Model file for the job. Use its own axes, mm. A direction names the side the tool comes from. Round coordinates to 2 decimals unless told otherwise and drop trailing zeros. Loops run counter-clockwise (first coordinate to the right, second up) from the corner with the lowest first, then second, coordinate; pieces in that order, holes last. Notation, with made-up numbers: (88, 9.5) - (143, 9.5) arc R10 cw to (143, 25.5) - close; hole circle Ø1 at (-25.5, 28.25). An arc over 180 degrees is marked (long way). Answer as a JSON object with one key per item and string values.
from build123d import *

# Parameters (mm, degrees)
F0_R     = 4.2591952999
F1_DEPTH = 2.286
F2_SIZE  = 1.016
F3_R     = 0.889
F4_SIZE  = 0.762
F5_SIZE  = 0.762


with BuildPart() as f1:
    # F0 (on Top) → F1 (new body)
    with BuildSketch(Plane.XY):
        Polygon((0, 14.6646975499), (-12.700000617, 21.9970463248), (-12.700000617, 7.3323487749), align=None)
        Polygon((12.700000617, 21.9970463248), (0, 14.6646975499), (12.700000617, 7.3323487749), align=None)
        Polygon((12.700000617, 7.3323487749), (0, 14.6646975499), (-12.700000617, 7.3323487749), (-12.700000617, -7.3323487749), (0, -14.6646975499), (12.700000617, -7.3323487749), align=None)
        Circle(F0_R, mode=Mode.SUBTRACT)
        Polygon((-12.700000617, -7.3323487749), (-12.700000617, 7.3323487749), (-25.400001234, 0), align=None)
        Polygon((-20.6551154208, 0), (-12.7952113226, 4.5379177469), (-12.7952113226, -4.5379177469), align=None, mode=Mode.SUBTRACT)
        Polygon((25.400001234, 0), (12.700000617, 7.3323487749), (12.700000617, -7.3323487749), align=None)
        Polygon((12.7952113226, -4.5379177469), (12.7952113226, 4.5379177469), (20.6551154208, 0), align=None, mode=Mode.SUBTRACT)
        Polygon((0, -14.6646975499), (-12.700000617, -7.3323487749), (-12.700000617, -21.9970463248), align=None)
        Polygon((12.700000617, -21.9970463248), (12.700000617, -7.3323487749), (0, -14.6646975499), align=None)
    extrude(amount=F1_DEPTH)

    # F2
    f2_edges = [f1.edges().sort_by_distance(p)[0] for p in [
        (-6.35, 18.330872, 2.286),
        (-12.700001, 14.664698, 2.286),
        (-19.050001, 3.666174, 2.286),
        (-19.050001, -3.666174, 2.286),
        (-12.700001, -14.664698, 2.286),
        (-6.35, -18.330872, 2.286),
        (6.35, -18.330872, 2.286),
        (12.700001, -14.664698, 2.286),
        (19.050001, -3.666174, 2.286),
        (19.050001, 3.666174, 2.286),
        (12.700001, 14.664698, 2.286),
        (6.35, 18.330872, 2.286),
    ]]
    chamfer(f2_edges, length=F2_SIZE)

    # F3
    f3_edges = [f1.edges().sort_by_distance(p)[0] for p in [
        (-4.259195, 0, 0),
        (-4.259195, 0, 2.286),
    ]]
    fillet(f3_edges, radius=F3_R)

    # F4
    f4_edges = [f1.edges().sort_by_distance(p)[0] for p in [
        (-6.35, -18.330872, 0),
        (6.35, -18.330872, 0),
        (12.700001, -14.664698, 0),
        (19.050001, -3.666174, 0),
        (19.050001, 3.666174, 0),
        (12.700001, 14.664698, 0),
        (6.35, 18.330872, 0),
        (-6.35, 18.330872, 0),
        (-12.700001, 14.664698, 0),
        (-19.050001, 3.666174, 0),
        (-19.050001, -3.666174, 0),
        (-12.700001, -14.664698, 0),
    ]]
    chamfer(f4_edges, length=F4_SIZE)

    # F5
    f5_edges = [f1.edges().sort_by_distance(p)[0] for p in [
        (-16.725163, 2.268959, 2.286),
        (-12.795211, 0, 2.286),
        (-16.725163, -2.268959, 2.286),
        (12.795211, 0, 2.286),
        (16.725163, 2.268959, 2.286),
        (16.725163, -2.268959, 2.286),
        (16.725163, 2.268959, 0),
        (12.795211, 0, 0),
        (16.725163, -2.268959, 0),
        (-16.725163, 2.268959, 0),
        (-16.725163, -2.268959, 0),
        (-12.795211, 0, 0),
    ]]
    chamfer(f5_edges, length=F5_SIZE)


solid = f1.part
1) Slice it at D-D on y = 19. List the corners of the cut face in (x, z), then the cut area to 3 significant figures.
Values follow:
{"outline": "(-12.7, 0.76) - (-11.94, 0) - (-9.03, 0) - (-7.51, 0.76) - (-7.51, 1.27) - (-9.54, 2.29) - (-11.68, 2.29) - (-12.7, 1.27) - close; (7.51, 0.76) - (9.03, 0) - (11.94, 0) - (12.7, 0.76) - (12.7, 1.27) - (11.68, 2.29) - (9.54, 2.29) - (7.51, 1.27) - close", "area": "18.9 mm²"}
2) Slice it at A-A on y = -18.5. List the corners of the cut face in (x, z), then the cut area to 3 significant figures.
Values follow:
{"outline": "(-12.7, 0.76) - (-11.94, 0) - (-8.17, 0) - (-6.64, 0.76) - (-6.64, 1.27) - (-8.67, 2.29) - (-11.68, 2.29) - (-12.7, 1.27) - close; (6.64, 0.76) - (8.17, 0) - (11.94, 0) - (12.7, 0.76) - (12.7, 1.27) - (11.68, 2.29) - (8.67, 2.29) - (6.64, 1.27) - close", "area": "22.9 mm²"}
3) Drop flat-ended pins along their axis: P1, Ø0.6, axis at y = -17, z = 1, coming from the -X side; P2, Ø1, axis at y = -6, z = 1, coming from the -X side. Give the stop position or say it passes through.
Values follow:
{"P1": "x = -12.7", "P2": "x = -15.87"}
4) Slice it at B-B on x = -6.5. List the corners of the cut face in (y, z), then the cut area to 3 significant figures.
Values follow:
{"outline": "(-18.42, 0.76) - (-17.54, 0) - (17.54, 0) - (18.42, 0.76) - (18.42, 1.27) - (17.24, 2.29) - (-17.24, 2.29) - (-18.42, 1.27) - close", "area": "82.3 mm²"}
5) Probe probe 1 along Y at (x, z) = (0, 1.05); probe 2 along X at (y, z) = (-3.5, 1.45); probe 3 along X at (y, z) = (-0.5, 1.5). List the from-to ranges inside material, lowest first.
Values follow:
{"probe 1": "-14.66 to -4.26, 4.26 to 14.66", "probe 2": "-18.98 to -14.59, -12.8 to -2.43, 2.43 to 12.8, 14.59 to 18.98", "probe 3": "-24.07 to -19.79, -12.8 to -4.24, 4.24 to 12.8, 19.79 to 24.07"}
6) Slice it at C-C on y = 10. List the corners of the cut face in (x, z).
Values follow:
{"outline": "(-12.7, 0.76) - (-11.94, 0) - (11.94, 0) - (12.7, 0.76) - (12.7, 1.27) - (11.68, 2.29) - (-11.68, 2.29) - (-12.7, 1.27) - close"}
7) Tool access for faces 1 (the flat face through (-6.256, 17.843, 0.386)), 2 (the flat face through (16.78, -2.237, 1.138)), 3 (the flat face through (16.99, -2.56, 1.91)), 4 (the flat face through (-16.98, 2.55, 0.39)): list every direction of +Z, -Z, +X, -X, +Y, -Y with a clear straight run to the whole face (end or side of a thin tool).
Values follow:
{"face 1": "-Z, +Y", "face 2": "+Z, -Z", "face 3": "+Z", "face 4": "-Z"}
8) Two-plate mould, pull along Y, no slides. Class faces 5 (the flat face through (-16.78, 2.237, 1.138)), 6 (the flat face through (-6.3, 18.3, 1)), 7 (the flat face through (-6, 0, 0)), 8 (the flat face through (18.58, -3.504, 0.386)): pulls with the +Y half, pulls with the -Y half, needs draft (parallel to the pull), parting line crosses it, or undercut.
Values follow:
{"face 5": "undercut", "face 6": "pulls with the +Y half", "face 7": "needs draft", "face 8": "pulls with the -Y half"}
